Autodesk Inventor part; units mm, degrees
ref_plane "YZ Plane" through (0, 0, 0) normal (1, 0, 0) x (0, 1, 0)
ref_plane "XZ Plane" through (0, 0, 0) normal (0, 1, 0) x (-1, 0, 0)
ref_plane "XY Plane" through (0, 0, 0) normal (0, 0, 1) x (1, 0, 0)
sketch "Sketch1" plane through (0, 0, 0) normal (0, 0, 1) x (1, 0, 0)
  line L0 (0, 0) -> (50.8, 0)
  line L1 (50.8, 0) -> (50.8, 355.6)
  line L2 (50.8, 355.6) -> (0, 355.6)
  line L3 (0, 355.6) -> (0, 0)
  dimension "d0" = 50.8
  dimension "d1" = 355.6
extrude "Extrusion1" add sketch "Sketch1" along normal blind 6.35
sketch "Sketch2" plane through (0, 0, 6.35) normal (0, 0, 1) x (1, 0, 0)
  line L0 (50.8, 0) -> (50.8, 355.6)
  line L1 (50.8, 152.4) -> (50.8, 203.2)
  line L2 (0, 152.4) -> (0, 203.2)
  line L3 (0, 355.6) -> (0, 0)
  line L4 (-88.9, 254) -> (0, 254)
  line L5 (0, 254) -> (0, 203.2)
  line L6 (0, 203.2) -> (-88.9, 203.2)
  line L7 (-88.9, 203.2) -> (-88.9, 254)
  line L8 (-88.9, 152.4) -> (0, 152.4)
  line L9 (0, 152.4) -> (0, 101.6)
  line L10 (0, 101.6) -> (-88.9, 101.6)
  line L11 (-88.9, 101.6) -> (-88.9, 152.4)
  line L12 (50.8, 101.6) -> (139.7, 101.6)
  line L13 (139.7, 101.6) -> (139.7, 152.4)
  line L14 (139.7, 152.4) -> (50.8, 152.4)
  line L15 (50.8, 152.4) -> (50.8, 101.6)
  line L16 (139.7, 203.2) -> (50.8, 203.2)
  line L17 (50.8, 203.2) -> (50.8, 254)
  line L18 (50.8, 254) -> (139.7, 254)
  line L19 (139.7, 254) -> (139.7, 203.2)
  point P0 (50.8, 152.4)
  point P1 (-88.9, 107.5788)
  point P2 (0, 254)
extrude "Extrusion3" add sketch "Sketch2" against normal blind 6.35
thicken "Thicken1" operation add thickness 101.6 both sides no extend neighbours yes toward (0, 1, 0) faces at (16.9333, 0, 2.1167)
thicken "Thicken2" operation add thickness 88.9 both sides no extend neighbours yes toward (-1, 0, 0) faces at (139.7, 220.1333, 2.1167)
thicken "Thicken3" operation add thickness 88.9 both sides no extend neighbours yes toward (1, 0, 0) faces at (-88.9, 237.0667, 2.1167)
sketch "Sketch3" plane through (0, 152.4, 0) normal (-1, 0, 0) x (0, 0, 1)
  line L0 (0, 203.2) -> (6.35, 203.2)
  line L1 (0, 0) -> (0, 203.2)
  line L2 (6.35, 0) -> (6.35, 203.2)
  line L3 (0, 203.2) -> (6.35, 203.2)
  line L4 (6.35, 203.2) -> (6.35, 152.4)
  line L5 (6.35, 152.4) -> (0, 152.4)
  line L6 (0, 152.4) -> (0, 203.2)
  point P0 (0, -152.4)
extrude "Extrusion4" add sketch "Sketch3" along normal blind 88.9
sketch "Sketch4" plane through (50.8, 152.4, 0) normal (1, 0, 0) x (0, 0, -1)
  line L0 (-6.35, 152.4) -> (-6.35, 203.2)
  line L1 (0, 152.4) -> (0, 0)
  line L2 (-6.35, 203.2) -> (0, 203.2)
  line L3 (0, 203.2) -> (0, 152.4)
  line L4 (0, 152.4) -> (-6.35, 152.4)
  line L5 (-6.35, 152.4) -> (-6.35, 203.2)
  point P0 (0, -152.4)
extrude "Extrusion5" add sketch "Sketch4" along normal blind 88.9
properties part number "backplatelift"
Read the model definition and answer for the solid it produces. Units are mm, in the model's axes. A direction names the side the tool comes from. Give positions to 0.01 mm unless a question says otherwise; leave off trailing zeros. Order: outer loops, then holes, each group sorted by start corner. A loop starts at its lowest first (then second) coordinate and runs counter-clockwise, first axis right, second up. Notation, with made-up numbers: (-35.75, 47.25) -> (-24.75, 47.25) arc R19 ccw to (-24.75, 66.25) -> close; hole circle Ø5 at (30, 6). An arc over 180 degrees is marked (long way). Write item = value, one per line.
1. A cutting plane is placed at C-C, the plane y = 222. Write down the section's boundary in (x, z).
Numbers:
outline = (0, 0) -> (50.8, 0) -> (50.8, 6.35) -> (0, 6.35) -> close
2. A cutting plane is placed at A-A, the plane x = 105. Write down the section's boundary in (y, z).
Numbers:
outline = (101.6, 0) -> (152.4, 0) -> (152.4, 6.35) -> (101.6, 6.35) -> close; (304.8, 0) -> (355.6, 0) -> (355.6, 6.35) -> (304.8, 6.35) -> close
3. Straight lines are drawn through the part: line 1 along Y through (x, z) = (67, 3); line 2 along X through (y, z) = (155, 4.5). For each, find the intervals that lie inside material, in ascending order.
Numbers:
line_1 = 101.6 to 152.4, 304.8 to 355.6
line_2 = 0 to 50.8
4. For faces 1 (the face through (-44, 304.8, 3)), 2 (the face through (-88.9, 127, 3)), 3 (the face through (96, 152.4, 3)), determine the directions among +Z, -Z, +X, -X, +Y, -Y from which every point of the face is accessible in a straight line to the end or side of a thin tool.
Numbers:
face_1 = +Z, -Z, -X
face_2 = +Z, -Z, -X, +Y, -Y
face_3 = +Z, -Z, +X
5. A cutting plane is placed at B-B, the plane z = 2.5. Write down the section's boundary in (x, y), and give its area (3 significant figures).
Numbers:
outline = (-88.9, 101.6) -> (139.7, 101.6) -> (139.7, 152.4) -> (50.8, 152.4) -> (50.8, 304.8) -> (139.7, 304.8) -> (139.7, 355.6) -> (-88.9, 355.6) -> (-88.9, 304.8) -> (0, 304.8) -> (0, 152.4) -> (-88.9, 152.4) -> close
area = 31,000 mm²
6. Given pin 1 (1.9 mm diameter, centred on y = 190.5, z = 4, fed in from -X); pin 2 (1.9 mm diameter, centred on y = 196, z = 3.5, fed in from +X), each flat-ended and moving along its own axis, determine where each tip first touches the part or whether it passes through.
Numbers:
pin_1 = 0
pin_2 = 50.8
